Source: CAD feature listing. Evaluate the final solid. Frame: model axes, mm. A direction names the side the tool comes from. Coordinates: 2 decimals unless noted, no trailing zeros. Order: outer loops, then holes, each group sorted by start corner. A loop starts at its lowest first (then second) coordinate and runs counter-clockwise, first axis right, second up.
```python
from build123d import *

# Parameters (mm, degrees)
SKETCH1_R           = 1.25
BOSS_EXTRUDE1_DEPTH = 5


with BuildPart() as part:
    # Sketch1 → Boss-Extrude1 (new body)
    with BuildSketch(Plane.XY):
        with BuildLine():
            Line((-14, 0), (-14, 35.752157845))
            ThreePointArc((-14, 35.752157845), (-24.124447597, 45.876605442), (-14, 56.001053039))
            Line((-14, 56.001053039), (14, 56.001053039))
            ThreePointArc((14, 56.001053039), (24.124447597, 45.876605442), (14, 35.752157845))
            Line((14, 35.752157845), (14, 0))
            ThreePointArc((14, 0), (0, -14), (-14, 0))
        make_face()
        with Locations((6.72, -6.72)):
            Circle(SKETCH1_R, mode=Mode.SUBTRACT)
        with Locations((-6.01, -5.66)):
            Circle(SKETCH1_R, mode=Mode.SUBTRACT)
        with Locations(Location((5.66, 6.01, 0), (0, 0, 180))):
            Circle(SKETCH1_R, mode=Mode.SUBTRACT)
        with Locations(Location((-6.72, 6.72, 0), (0, 0, 180))):
            Circle(SKETCH1_R, mode=Mode.SUBTRACT)
    extrude(amount=BOSS_EXTRUDE1_DEPTH)


solid = part.part
```
Q1. Pull-direction query (X, two-part tool) for faces 1 (the flat face through (0, 56.001, 2)), 2 (the cylindrical face through (7.875, -7.199, 2.465)), 3 (the cylindrical face through (-24.12, 45.65, 2.46)), 4 (the cylindrical face through (-7.91, 6.34, 2.46)); classes: pulls with the +X half, pulls with the -X half, needs draft (parallel to the pull), parting line crosses it, or undercut.
Solutions:
face 1: needs draft
face 2: undercut
face 3: pulls with the -X half
face 4: undercut
Q2. Material intervals for line 1 along Y through (x, z) = (-6.72, 1.9); line 2 along Y through (x, z) = (-6.01, 3.2); line 3 along X through (y, z) = (6.01, 2.3), sorted ascending.
Solutions:
line 1: y = -12.28 to -6.69, -4.63 to 5.47, 7.97 to 56
line 2: y = -12.64 to -6.91, -4.41 to 5.69, 7.75 to 56
line 3: x = -14 to -7.75, -5.69 to 4.41, 6.91 to 14
Q3. Set-up query: faces 5 (the flat face through (-14, 18, 2)), 6 (the flat face through (0, 29, 0)), 7 (the flat face through (14, 18, 2)). Return all of +Z, -Z, +X, -X, +Y, -Y with unobstructed straight access to the full face (end or side cutting, diameter ignored); none if empty.
Solutions:
face 5: +Z, -Z, -X, -Y
face 6: -Z, +X, -X, +Y, -Y
face 7: +Z, -Z, +X, -Y
Q4. Pin query (flat end, axial travel): P1, Ø3, axis at x = 6.72, y = -6.72, coming from the +Z side; P2, Ø2.5, axis at y = 10.5, z = 2, coming from the -X side. Return the tip coordinate at first contact, or that it passes through.
Solutions:
P1: stops at z = 5
P2: stops at x = -14
Q5. Section query B-B on y = 1. Output: boundary loops of the cut face in (x, z), plus the area to 3 significant figures.
Solutions:
outline: (-14, 0) - (14, 0) - (14, 5) - (-14, 5) - close
area: 140 mm2
Q6. Section query C-C on y = 51.5. Output: boundary loops of the cut face in (x, z), plus the area to 3 significant figures.
Solutions:
outline: (-22.42, 0) - (22.42, 0) - (22.42, 5) - (-22.42, 5) - close
area: 224 mm2
Q7. Section query A-A on z = 3.7. Output: boundary loops of the cut face in (x, y), plus the area to 3 significant figures.
Solutions:
outline: (-14, 0) arc R14 ccw to (14, 0) - (14, 35.75) arc R10.12 ccw to (14, 56) - (-14, 56) arc R10.12 ccw to (-14, 35.75) - close; hole circle Ø2.5 at (-6.72, 6.72); hole circle Ø2.5 at (-6.01, -5.66); hole circle Ø2.5 at (5.66, 6.01); hole circle Ø2.5 at (6.72, -6.72)
area: 2,180 mm2
